Source: CAD feature listing. Evaluate the final solid. Frame: model axes, mm. Give positions to 0.01 mm unless a question says otherwise; leave off trailing zeros. Loops run counter-clockwise (first coordinate to the right, second up) from the corner with the lowest first, then second, coordinate; pieces in that order, holes last. Notation, with made-up numbers: (63, -7) -> (87, -7) arc R22 ccw to (87, 12) -> close; hole circle Ø2 at (47, -16.5). An arc over 180 degrees is marked (long way). Put each result on its own line as item: value.
```python
from build123d import *

# Parameters (mm, degrees)
F1_DEPTH = 3
F2_SIZE  = 9.525
F4_DEPTH = 0.7493
F6_D     = 9.525
F8_D     = 31.75
F9_R     = 2.54


# Not quite as in the source:
# - a length typed as a fraction of an inch, garbled in the dataset ("3 / 203.2 mm" for 3/8 in), is restored


with BuildPart() as f1:
    # F0 (on Top) → F1 (new body)
    with BuildSketch(Plane.XY):
        with BuildLine():
            Line((197.5066929404, 463.55), (0, 0))
            Line((0, 0), (971.55, 0))
            Line((971.55, 0), (971.55, 43.18))
            Line((971.55, 43.18), (1101.00364, 43.18))
            ThreePointArc((1101.00364, 43.18), (1100.0520555905, 255.6158899642), (1056.5397729404, 463.55))
            Line((1056.5397729404, 463.55), (197.5066929404, 463.55))
        make_face()
    extrude(amount=F1_DEPTH)

    # F2
    f2_edges = [f1.edges().sort_by_distance(p)[0] for p in [
        (971.55, 0, 1.5),
    ]]
    chamfer(f2_edges, length=F2_SIZE)

    # F3 (on face) → F4 (cut)
    with BuildSketch(Plane.XY.offset(3)):
        with BuildLine():
            Line((0, 0), (793.26486, 0))
            Line((793.26486, 0), (793.26486, 451.36562))
            Line((793.26486, 451.36562), (794.85236, 451.36562))
            Line((794.85236, 451.36562), (794.85236, 0))
            Line((794.85236, 0), (962.025, 0))
            Line((962.025, 0), (971.55, 9.525))
            Line((971.55, 9.525), (971.55, 43.18))
            Line((971.55, 43.18), (1101.00364, 43.18))
            ThreePointArc((1101.00364, 43.18), (1100.0520555905, 255.6158899642), (1056.5397729404, 463.55))
            Line((1056.5397729404, 463.55), (197.5066929404, 463.55))
            Line((197.5066929404, 463.55), (0, 0))
        make_face()
    extrude(amount=-F4_DEPTH, mode=Mode.SUBTRACT)

    # F6 (through all)
    with Locations(Plane.XY.offset(2.2507)):
        with Locations((209.7413209615, 445.0286267957), (409.2329209615, 445.516), (669.1511209615, 446.151), (113.7415553228, 219.7163059861), (28.5242, 19.7104), (262.7122, 20.176624196), (511.8862, 20.6726826953), (691.9722, 21.0312)):
            Hole(F6_D / 2)

    # F8 (through all)
    with Locations(Plane.XY.offset(2.2507)):
        with Locations((238.9469804498, 371.2718)):
            Hole(F8_D / 2)

    # F9
    f9_edges = [f1.edges().sort_by_distance(p)[0] for p in [
        (197.506693, 463.55, 1.12535),
        (1056.539773, 463.55, 1.12535),
        (1101.00364, 43.18, 1.12535),
        (971.55, 43.18, 1.12535),
        (971.55, 9.525, 1.12535),
        (962.025, 0, 1.12535),
        (0, 0, 1.12535),
    ]]
    fillet(f9_edges, radius=F9_R)


solid = f1.part
```
(1) First-contact query: P1, Ø8.5, axis at x = 669.15, y = 446.15, coming from the -Z side; P2, Ø12, axis at x = 604.5, y = 287.5, coming from the +Z side. Flat tips, straight axial feed; report the tip coordinate or a pass-through.
Calculated:
P1: passes through
P2: stops at z = 2.25
(2) Line query: probe 1 along Y at (x, z) = (263, 0.75); probe 2 along Y at (x, z) = (261.5, 0.35); probe 3 along Z at (x, y) = (798, 125). Output: solid intervals per line, ascending. Write a range as from..to.
Calculated:
probe 1: y = 0..15.42, 24.93..463.55
probe 2: y = 0..15.57, 24.78..463.55
probe 3: z = 0..2.25
(3) Section A-A on y = 330. Return loops of the section in (x, z), then the cut area to 3 significant figures.
Calculated:
outline: (140.6, 0) -> (1089.49, 0) -> (1089.49, 2.25) -> (794.85, 2.25) -> (794.85, 3) -> (793.26, 3) -> (793.26, 2.25) -> (140.6, 2.25) -> close
area: 2,140 mm²
(4) Draft query along X for faces 1 (the flat face through (100.545, 235.98, 1.11)), 2 (the cylindrical face through (1100.335, 252.905, 1.11)), 3 (the flat face through (546, 235, 0)), 4 (the cylindrical face through (231.6, 357.2, 1.1)). Return one class per face: released by +X, released by -X, zero draft, split by the parting line, or undercut.
Calculated:
face 1: released by -X
face 2: released by +X
face 3: zero draft
face 4: undercut
(5) Section C-C on x = 496. Return loops of the section in (y, z).
Calculated:
outline: (0, 0) -> (463.55, 0) -> (463.55, 2.25) -> (0, 2.25) -> close
(6) Section B-B on z = 0.65. Give the number of separate pieces and of enclosed holes in the cut face, then the cut area to 3 significant figures.
Calculated:
separate pieces: 1
enclosed holes: 9
area: 454,000 mm²
(7) Section D-D on y = 95. Return loops of the section in (x, z).
Calculated:
outline: (40.48, 0) -> (1104.73, 0) -> (1104.73, 2.25) -> (794.85, 2.25) -> (794.85, 3) -> (793.26, 3) -> (793.26, 2.25) -> (40.48, 2.25) -> close
